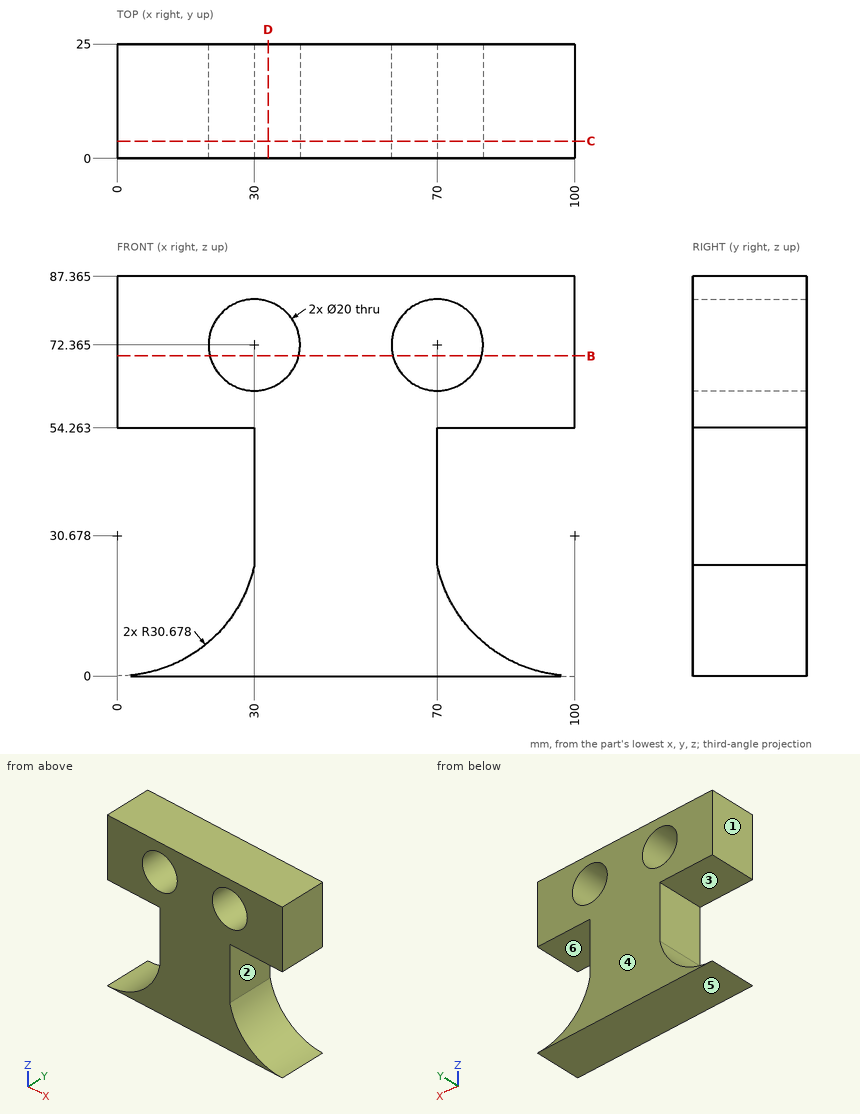
Input: dimensioned drawing with shaded views. Units: mm. Origin: part minimum x, y, z. A direction names the side the tool comes from. Round coordinates to 2 decimals unless told otherwise and drop trailing zeros. Order: outer loops, then holes, each group sorted by start corner. A loop starts at its lowest first (then second) coordinate and runs counter-clockwise, first axis right, second up. Notation, with made-up numbers: (56.5, 76.5) -> (65.5, 76.5) arc R18 cw to (65.5, 92.5) -> close; hole circle Ø4 at (77.5, 47.25). An arc over 180 degrees is marked (long way). Put each result on its own line as item: value. Start each with the question number.
Q1. Section B-B on z = 70. Return the cut outline in (x, y).
Q2. First-contact query: pin 1 (16 mm diameter, centred on x = 70, z = 72.36, fed in from +Y); pin 2 (12.5 mm diameter, centred on y = 13.5, z = 37.5, fed in from -X); pin 3 (1.5 mm diameter, centred on y = 6, z = 21.5, fed in from +X); pin 4 (1.5 mm diameter, centred on y = 6.5, z = 49, fed in from +X). Flat tips, straight axial feed; report the tip coordinate or a pass-through.
Q3. Section C-C on y = 3.75. Return the cut outline in (x, z) (1 decimal).
Q4. Line query: probe 1 along X at (y, z) = (4.5, 65.5); probe 2 along X at (y, z) = (14, 48.5); probe 3 along X at (y, z) = (12.5, 79.5) (1 decimal). Output: solid intervals per line, ascending.
Q5. Section D-D on x = 33. Return the cut outline in (y, z) (1 decimal), and give its area (3 significant figures).
Q6. Pull-direction query (Z, two-part tool) for the marked faces 4, 5 and 6; classes: +Z half, -Z half, draft (parallel to the pull), parting line (faces both ways), or undercut.
Q7. Reachability of the marked faces 1, 2 and 3 from +Z, -Z, +X, -X, +Y, -Y: full face, straight path, thin tool, end or side. Return the list, or none.
Ans:
1. outline: (0, 0) -> (20.28, 0) -> (20.28, 25) -> (0, 25) -> close; (39.72, 0) -> (60.28, 0) -> (60.28, 25) -> (39.72, 25) -> close; (79.72, 0) -> (100, 0) -> (100, 25) -> (79.72, 25) -> close
2. pin 1: passes through
2. pin 2: stops at x = 30
2. pin 3: stops at x = 70.97
2. pin 4: stops at x = 70
3. outline: (0, 0) -> (100, 0) arc R30.7 cw to (70, 24.3) -> (70, 54.3) -> (100, 54.3) -> (100, 87.4) -> (0, 87.4) -> (0, 54.3) -> (30, 54.3) -> (30, 24.3) arc R30.7 cw to start; hole circle Ø20 at (30, 72.4); hole circle Ø20 at (70, 72.4)
4. probe 1: x = 0 to 22.73, 37.27 to 62.73, 77.27 to 100
4. probe 2: x = 30 to 70
4. probe 3: x = 0 to 23, 37 to 63, 77 to 100
5. outline: (0, 0) -> (25, 0) -> (25, 62.8) -> (0, 62.8) -> close; (0, 81.9) -> (25, 81.9) -> (25, 87.4) -> (0, 87.4) -> close
5. area: 1,710 mm2
6. face 4: draft
6. face 5: -Z half
6. face 6: undercut
7. face 1: +Z, -Z, -X, +Y, -Y
7. face 2: +X, +Y, -Y
7. face 3: -X, +Y, -Y
